Verification items for the finished model (mm, model axes). Face numbers are marked on the shaded views. Give positions to 0.01 mm unless a question says otherwise; leave off trailing zeros. Order: outer loops, then holes, each group sorted by start corner. A loop starts at its lowest first (then second) coordinate and runs counter-clockwise, first axis right, second up. Notation, with made-up numbers: (51, 63) -> (55, 63) arc R25 ccw to (55, 92) -> close; hole circle Ø11 at (50, -24). An arc over 180 degrees is marked (long way). Return JSON: item names as keys, results as strings. Group by question number.
(1) Release check for a two-part mould opening along X. For the marked faces 1, 2 and 3 record: pulls with the +X half, pulls with the -X half, needs draft (parallel to the pull), parting line crosses it, or undercut.
(2) Cross-section at C-C on y = 5.5. Enter the section's corners in (x, z).
(3) Thickness scan on line 1 along Z through (x, y) = (-70.5, 2); line 2 along X through (y, z) = (12.25, -71); line 3 along X through (y, z) = (1, -72.5). Record the ranges inside material, lowest first.
(4) Cross-section at B-B on y = 9.75. Enter the section's corners in (x, z), then the cut area to 3 significant figures.
(5) Cross-section at D-D on z = -53.75. Enter the section's corners in (x, y).
(6) Cross-section at A-A on z = -70.75. Enter the section's corners in (x, y).
(7) Depth check by flat-ended pin: pin 1 Ø1.5 at (x, y) = (-70, 9.5) entering from +Z. Enter the tip coordinate at first touch or a pass-through.
from build123d import *

# Parameters (mm, degrees)
SKETCH1_W           = 25
SKETCH1_H           = 5.842
BOSS_EXTRUDE1_DEPTH = 15
SKETCH5_R           = 2.54
CUT_EXTRUDE3_DEPTH  = 85.289149032
SKETCH7_R           = 3.302
CUT_EXTRUDE4_DEPTH  = 1.27
SKETCH10_R          = 1.0795
CUT_EXTRUDE7_DEPTH  = 102.459910937
SKETCH11_W          = 25
SKETCH11_H          = 15
BOSS_EXTRUDE2_DEPTH = 20
SKETCH12_R          = 1.75
CUT_EXTRUDE8_DEPTH  = 114.864732767


with BuildPart() as part:
    # Sketch1 → Boss-Extrude1 (new body)
    with BuildSketch(Plane(origin=(0, 0, 0), x_dir=(1, 0, 0), z_dir=(0, 1, 0))):
        with Locations((-70.237728278, 53.855595943)):
            Rectangle(SKETCH1_W, SKETCH1_H)
    extrude(amount=BOSS_EXTRUDE1_DEPTH)

    # Sketch5 → Cut-Extrude3 (cut, through all)
    with BuildSketch(Plane.XY.offset(-50.934595943)):
        with Locations((-70.237728278, 8.396)):
            Circle(SKETCH5_R)
    extrude(amount=-CUT_EXTRUDE3_DEPTH, mode=Mode.SUBTRACT)

    # Sketch7 → Cut-Extrude4 (cut)
    with BuildSketch(Plane.XY.offset(-50.934595943)):
        with Locations((-70.237728278, 8.396)):
            Circle(SKETCH7_R)
    extrude(amount=-CUT_EXTRUDE4_DEPTH, mode=Mode.SUBTRACT)

    # Sketch10 → Cut-Extrude7 (cut, through all)
    with BuildSketch(Plane(origin=(0, 15, 0), x_dir=(1, 0, 0), z_dir=(0, 1, 0))):
        with Locations(Location((-70.237728278, 53.982595943, 0), (0, 0, 270))):
            Circle(SKETCH10_R)
    extrude(amount=-CUT_EXTRUDE7_DEPTH, mode=Mode.SUBTRACT)

    # Sketch11 → Boss-Extrude2 (add)
    with BuildSketch(Plane(origin=(0, 0, -56.776595943), x_dir=(-1, 0, 0), z_dir=(0, 0, -1))):
        with Locations((70.237728278, 7.5)):
            Rectangle(SKETCH11_W, SKETCH11_H)
    extrude(amount=BOSS_EXTRUDE2_DEPTH)

    # Sketch12 → Cut-Extrude8 (cut, through all)
    with BuildSketch(Plane(origin=(0, 15, 0), x_dir=(1, 0, 0), z_dir=(0, 1, 0))):
        with Locations(Location((-70.237728278, 71.776595943, 0), (0, 0, 270))):
            Circle(SKETCH12_R)
    extrude(amount=-CUT_EXTRUDE8_DEPTH, mode=Mode.SUBTRACT)


solid = part.part
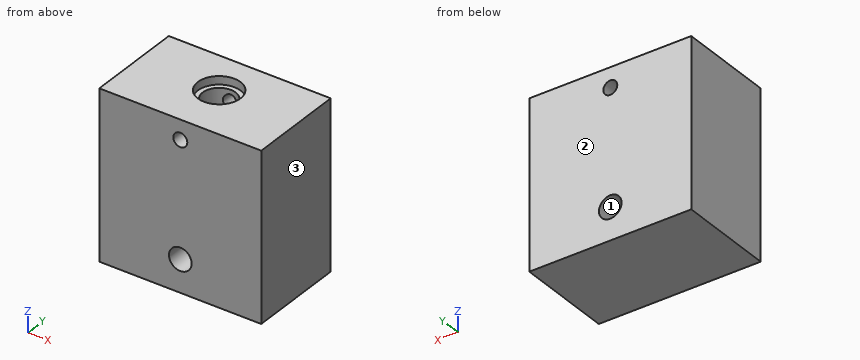
Verdict:
{
 "1": {"face 1": "undercut", "face 2": "needs draft", "face 3": "pulls with the +X half"},
 "2": {"outline": "(-82.74, -76.78) -> (-57.74, -76.78) -> (-57.74, -50.93) -> (-68.65, -50.93) -> (-68.65, -52.2) -> (-71.82, -52.2) -> (-71.82, -50.93) -> (-82.74, -50.93) -> close; hole circle Ø3.5 at (-70.24, -71.78); hole circle Ø2.16 at (-70.24, -53.98)"},
 "3": {"line 1": "-76.78 to -73.51, -70.05 to -55.03, -52.94 to -50.93", "line 2": "-82.74 to -71.81, -68.67 to -57.74", "line 3": "-82.74 to -71.83, -68.64 to -57.74"},
 "4": {"outline": "(-82.74, -76.78) -> (-57.74, -76.78) -> (-57.74, -50.93) -> (-67.23, -50.93) -> (-67.23, -52.2) -> (-68.09, -52.2) -> (-68.09, -56.78) -> (-72.39, -56.78) -> (-72.39, -52.2) -> (-73.25, -52.2) -> (-73.25, -50.93) -> (-82.74, -50.93) -> close; hole circle Ø3.5 at (-70.24, -71.78)", "area": "609 mm²"},
 "5": {"outline": "(-82.74, 0) -> (-71.29, 0) -> (-71.29, 6.09) arc R2.54 cw to (-71.29, 10.71) -> (-71.29, 15) -> (-82.74, 15) -> close; (-69.18, 0) -> (-57.74, 0) -> (-57.74, 15) -> (-69.18, 15) -> (-69.18, 10.71) arc R2.54 cw to (-69.18, 6.09) -> close"},
 "6": {"outline": "(-82.74, 0) -> (-71.65, 0) -> (-71.65, 15) -> (-82.74, 15) -> close; (-68.82, 0) -> (-57.74, 0) -> (-57.74, 15) -> (-68.82, 15) -> close"},
 "7": {"pin 1": "z = -56.78"}
}
